Autodesk Inventor part; units mm, degrees
ref_plane "YZ Plane" through (0, 0, 0) normal (1, 0, 0) x (0, 1, 0)
ref_plane "XZ Plane" through (0, 0, 0) normal (0, 1, 0) x (-1, 0, 0)
ref_plane "XY Plane" through (0, 0, 0) normal (0, 0, 1) x (1, 0, 0)
sketch "Boceto1" plane through (0, 0, 0) normal (0, 1, 0) x (-1, 0, 0)
  line L0 (-20, 20) -> (-20, -20)
  line L1 (20, -20) -> (20, 20)
  arc A0 (20, 40) -> (-20, 40) centre (0, 40) ccw
  arc A1 (-20, -40) -> (20, -40) centre (0, -40) ccw
  circle A2 centre (0, -40) radius 10
  line L2 (20, 20) -> (20, 40)
  line L3 (-20, 20) -> (-20, 40)
  line L4 (20, -20) -> (20, -40)
  line L5 (-20, -20) -> (-20, -40)
  circle A3 centre (0, 40) radius 10
  point P0 (0, 0)
extrude "Extrusión1" add sketch "Boceto1" along normal blind 10
sketch "Boceto2" plane through (20, 0, 40) normal (1, 0, 0) x (0, 0, -1)
  line L0 (80, 10) -> (0, 10) construction
  circle A0 centre (40, 30) radius 10
  arc A1 (60, 30) -> (20, 30) centre (40, 30) ccw
  line L1 (20, 30) -> (20, 10)
  line L2 (60, 30) -> (60, 10)
  line L3 (20, 10) -> (60, 10)
  point P0 (40, 0)
extrude "Extrusión2" add sketch "Boceto2" against normal blind 40
thread "Rosca1"
thread "Rosca2"
thread "Rosca3"
properties part number "Tarea 1 Lab Dinamica"
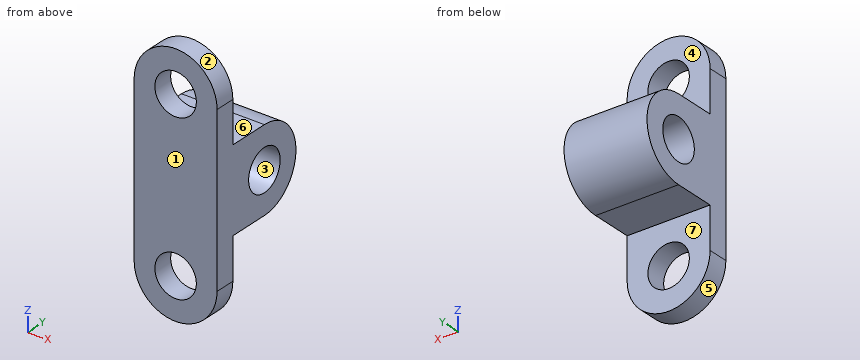
Part model, mm, in its own coordinate system. Face numbers are marked on the shaded views. A direction names the side the tool comes from. Coordinates: 2 decimals unless noted, no trailing zeros. Loops run counter-clockwise (first coordinate to the right, second up) from the corner with the lowest first, then second, coordinate; pieces in that order, holes last. Notation, with made-up numbers: (53, 44.5) - (88, 44.5) arc R20 cw to (88, 80.5) - close; hole circle Ø1 at (73, 53.25). An arc over 180 degrees is marked (long way). Write item = value, one per line. Start each with the question number.
Item 1: 3-axis set-ups, long thin cutter, end or side, ignore diameter. For the marked faces 5, 6 and 7: which of +Z, -Z, +X, -X, +Y, -Y reach the whole face in a straight line?
Item 2: Cut at A-A, the plane x = 0. Give the cut face in (y, z).
Item 3: Cut at D-D, the plane y = 15.5. Give the cut face in (x, z).
Item 4: Mould opens along Y. For the marked faces 1, 2, 3 and 4 say: released by +Y, released by -Y, zero draft, split by the parting line, or undercut.
Item 5: Flat gauge pins, fed straight in: pin 1 Ø1.5 at (x, y) = (3, 31.5) entering from +Z; pin 2 Ø12 at (x, z) = (2, -46.5) entering from +Y; pin 3 Ø8 at (x, y) = (-2.5, 43.5) entering from +Z; pin 4 Ø16 at (x, z) = (0, -40) entering from +Y (3 decimals). Where does each tip first touch, or does it go through?
Item 6: Cut at C-C, the plane x = -16.5. Give the cut face in (y, z).
Item 7: Cut at B-B, the plane z = 0. Give the cut face in (x, y), and give its area (3 significant figures).
Item 8: Wall check: L1, parallel to Z at x = -4, y = 6.5; L2, parallel to Z at x = 0, y = 5; L3, parallel to Y at x = -7, z = 0. Give the ranges that are in metal, low to high. Write a range as from..to.
The answers:
q1.face_5 = -Z, +Y, -Y
q1.face_6 = +Z, +X, -X, +Y
q1.face_7 = -Z, +X, -X, +Y
q2.outline = (0, -60) - (10, -60) - (10, -50) - (0, -50) - close; (0, -30) - (10, -30) - (10, -20) - (30, -20) arc R20 ccw to (30, 20) - (10, 20) - (10, 30) - (0, 30) - close; (0, 50) - (10, 50) - (10, 60) - (0, 60) - close; hole circle Ø20 at (30, 0)
q3.outline = (-20, -20) - (20, -20) - (20, 20) - (-20, 20) - close
q4.face_1 = released by -Y
q4.face_2 = zero draft
q4.face_3 = undercut
q4.face_4 = released by +Y
q5.pin_1 = 19.99
q5.pin_2 = 10
q5.pin_3 = 17.6
q5.pin_4 = through
q6.outline = (0, -51.3) - (10, -51.3) - (10, -20) - (30, -20) arc R20 ccw to (30, 20) - (10, 20) - (10, 51.3) - (0, 51.3) - close; hole circle Ø20 at (30, 0)
q7.outline = (-20, 0) - (20, 0) - (20, 20) - (-20, 20) - close; (-20, 40) - (20, 40) - (20, 50) - (-20, 50) - close
q7.area = 1,200 mm2
q8.L1 = -59.6..-49.17, -30.83..30.83, 49.17..59.6
q8.L2 = -60..-50, -30..30, 50..60
q8.L3 = 0..20, 40..50
